```python
from build123d import *

# Parameters (mm, degrees)
F0_R     = 1.7
F1_DEPTH = 3
F2_R     = 2
F3_R     = 1.7
F4_DEPTH = 6
F5_R     = 2
F6_R     = 1.7
F7_DEPTH = 3
F8_R     = 2.9
F9_DEPTH = 1.5


with BuildPart() as f1:
    # F0 (on Top) → F1 (new body)
    with BuildSketch(Plane.XY):
        Polygon((-2.5, 2.5), (-2.5, 0), (-2.5, -2.5), (58.5, -2.5), (58.5, 0), (58.5, 2.5), align=None)
        Circle(F0_R, mode=Mode.SUBTRACT)
        with Locations((56, 0)):
            Circle(F0_R, mode=Mode.SUBTRACT)
    extrude(amount=F1_DEPTH)

    # F2
    f2_edges = [f1.edges().sort_by_distance(p)[0] for p in [
        (-2.5, 2.5, 1.5),
        (-2.5, -2.5, 1.5),
        (58.5, 2.5, 1.5),
        (58.5, -2.5, 1.5),
    ]]
    fillet(f2_edges, radius=F2_R)

    # F3 (on face) → F4 (join)
    with BuildSketch(Plane(origin=(0, 0, 0), x_dir=(1, 0, 0), z_dir=(0, 0, -1))):
        with BuildLine():
            Line((53.5, -2.5), (56.5, -2.5))
            ThreePointArc((56.5, -2.5), (57.9142135624, -1.9142135624), (58.5, -0.5))
            Line((58.5, -0.5), (58.5, 0.5))
            ThreePointArc((58.5, 0.5), (57.9142135624, 1.9142135624), (56.5, 2.5))
            Line((56.5, 2.5), (53.5, 2.5))
            Line((53.5, 2.5), (53.5, -2.5))
        make_face()
        with Locations((56, 0)):
            Circle(F3_R, mode=Mode.SUBTRACT)
    extrude(amount=F4_DEPTH)

    # F5
    f5_edges = [f1.edges().sort_by_distance(p)[0] for p in [
        (53.5, 2.5, -3),
        (53.5, -2.5, -3),
    ]]
    fillet(f5_edges, radius=F5_R)

    # F6 (on face) → F7 (join, through all)
    with BuildSketch(Plane.XY.offset(3)):
        with BuildLine():
            ThreePointArc((-0.5, 3.5), (-2.6213203436, 2.6213203436), (-3.5, 0.5))
            Line((-3.5, 0.5), (-3.5, -0.5))
            ThreePointArc((-3.5, -0.5), (-2.6213203436, -2.6213203436), (-0.5, -3.5))
            Line((-0.5, -3.5), (3, -3.5))
            Line((3, -3.5), (3, -2.5))
            Line((3, -2.5), (3, 2.5))
            Line((3, 2.5), (3, 3.5))
            Line((3, 3.5), (-0.5, 3.5))
        make_face()
        Circle(F6_R, mode=Mode.SUBTRACT)
    extrude(amount=-F7_DEPTH)

    # F8 (on face) → F9 (cut)
    with BuildSketch(Plane(origin=(0, 0, 0), x_dir=(1, 0, 0), z_dir=(0, 0, -1))):
        Circle(F8_R)
    extrude(amount=-F9_DEPTH, mode=Mode.SUBTRACT)


solid = f1.part
```
Part model, mm, in its own coordinate system. A direction names the side the tool comes from. Coordinates: 2 decimals unless noted, no trailing zeros. Write each loop counter-clockwise with the first axis right and the second up, starting at its lowest first coordinate (ties: lowest second). Pieces come first, ordered by that corner, then holes.
Item 1: Mould opens along X. For faces 1 (the face through (58.5, 0, -1)), 2 (the face through (-0.37, -1.66, 2.24)), 3 (the face through (32, -2.5, 1)) say: released by +X, released by -X, zero draft, split by the parting line, or undercut.
Item 2: Slice it at A-A (x = 37). Write the cut outline in (y, z).
Item 3: Pin check, flat tips, straight feed: pin 1 (0.8 mm diameter, centred on y = 0, z = -4, fed in from -X); pin 2 (1.5 mm diameter, centred on y = -2.5, z = -3.5, fed in from +X); pin 3 (2.5 mm diameter, centred on x = 56, y = 0, fed in from -Z); pin 4 (1 mm diameter, centred on x = 11.5, y = -1, fed in from -Z). Stop position of each tip, or through.
Item 4: Probe line 1 (X direction, y = 0, z = 0.65); line 2 (Y direction, x = 56, z = -2.5); line 3 (Y direction, x = 0, z = 2.55). List the from-to ranges inside material, lowest first.
Item 5: Which spindle directions (+Z, -Z, +X, -X, +Y, -Y) get a long thin tool onto all of the face, cutting with end or side? Do faces 4 (the face through (0, 2, 1.5)), 5 (the face through (3, -3, 2)), 6 (the face through (54.1, 1.93, -3.04)), 7 (the face through (53.5, 0, -3)), 8 (the face through (3, 3, 2)). Say none if no direction does.
Results found:
1. face 1: released by +X
1. face 2: undercut
1. face 3: zero draft
2. outline: (-2.5, 0) - (2.5, 0) - (2.5, 3) - (-2.5, 3) - close
3. pin 1: stops at x = 53.5
3. pin 2: stops at x = 58.06
3. pin 3: passes through
3. pin 4: stops at z = 0
4. line 1: x = -3.5 to -2.9, 2.9 to 54.3, 57.7 to 58.5
4. line 2: y = -2.5 to -1.7, 1.7 to 2.5
4. line 3: y = -3.5 to -1.7, 1.7 to 3.5
5. face 4: -Z
5. face 5: +Z, -Z, +X, -Y
5. face 6: -Z, -X, +Y
5. face 7: -Z, -X, +Y, -Y
5. face 8: +Z, -Z, +X, +Y
